Verification items for this drawing (mm, ordinates from the low corner). A direction names the side the tool comes from. Round coordinates to 2 decimals unless told otherwise and drop trailing zeros. Loops run counter-clockwise (first coordinate to the right, second up) from the corner with the lowest first, then second, coordinate; pieces in that order, holes last. Notation, with made-up numbers: (-38, -2) - (17, -2) arc R21 ccw to (17, 36) - close; hole circle Ø3 at (37, -21). An arc over 180 degrees is marked (long way). Put each result on its own line as item: value.
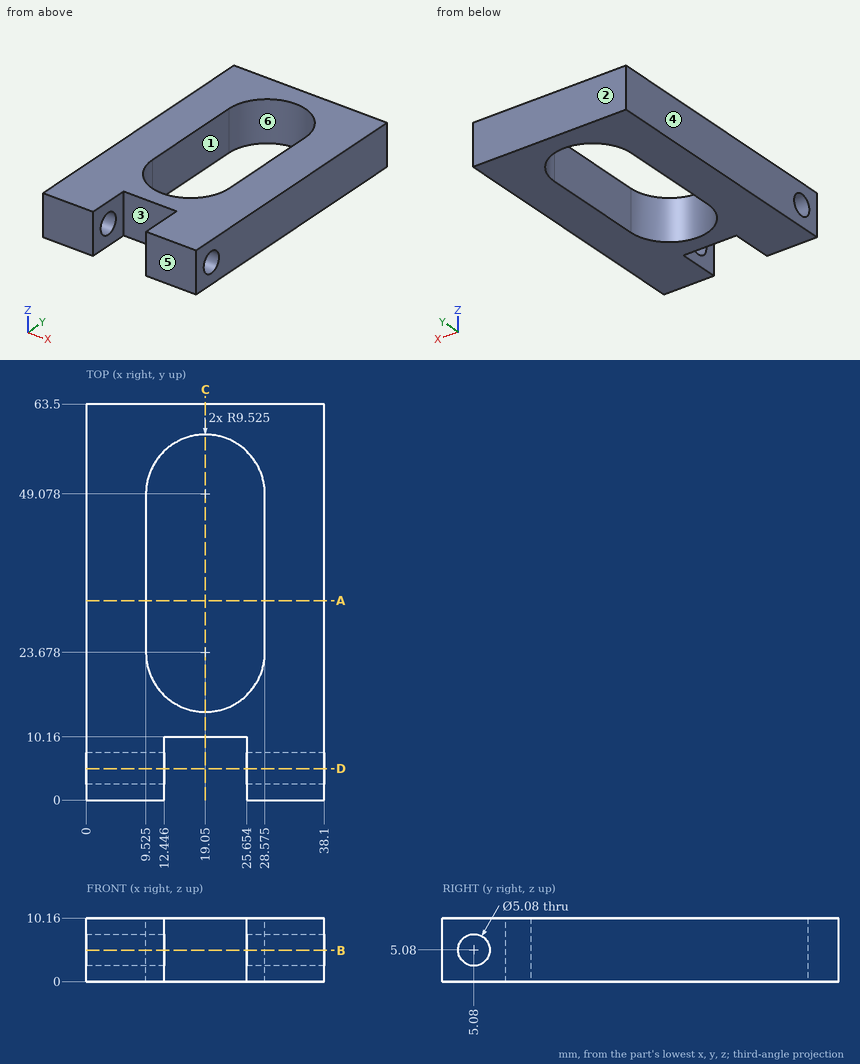
Item 1: Thickness scan on line 1 (X direction, y = 44.5, z = 4) (1 decimal); line 2 (Y direction, x = 27.5, z = 6.75) (1 decimal); line 3 (Y direction, x = 2.5, z = 5.25) (1 decimal). Record the ranges inside material, lowest first. Write a range as from..to.
Filled sheet:
line 1: 0..9.5, 28.6..38.1
line 2: 0..3.2, 7..19.3, 53.5..63.5
line 3: 0..2.5, 7.6..63.5
Item 2: Section check D-D on y = 5.08. Enter the section's corners in (x, z).
Filled sheet:
outline: (0, 0) - (12.45, 0) - (12.45, 2.54) - (0, 2.54) - close; (0, 7.62) - (12.45, 7.62) - (12.45, 10.16) - (0, 10.16) - close; (25.65, 0) - (38.1, 0) - (38.1, 2.54) - (25.65, 2.54) - close; (25.65, 7.62) - (38.1, 7.62) - (38.1, 10.16) - (25.65, 10.16) - close
Item 3: Section check A-A on y = 32. Enter the section's corners in (x, z) (1 decimal).
Filled sheet:
outline: (0, 0) - (9.5, 0) - (9.5, 10.2) - (0, 10.2) - close; (28.6, 0) - (38.1, 0) - (38.1, 10.2) - (28.6, 10.2) - close
Item 4: Tool access check on the marked faces 1, 2 and 3. Record the directions out of +Z, -Z, +X, -X, +Y, -Y that give a thin tool (end or side, any length) a straight path to the whole face; none if there is none.
Filled sheet:
face 1: +Z, -Z
face 2: +Z, -Z, +X, -X, +Y
face 3: +Z, -Z, -Y
Item 5: Go/stop test with a flat-tipped pin: pin 1 (1 mm diameter, centred on x = 13, z = 8.5, fed in from -Y). Record where the tip stops, or that it passes through.
Filled sheet:
pin 1: y = 10.16
Item 6: Release check for a two-part mould opening along Y. For the marked faces 4, 5 and 6 record: +Y half, -Y half, draft (parallel to the pull), parting line (faces both ways), or undercut.
Filled sheet:
face 4: draft
face 5: -Y half
face 6: undercut
Item 7: Section check B-B on z = 5. Count the separate pieces of the cut face and the enclosed holes in it, then the cut area to 3 significant figures.
Filled sheet:
separate pieces: 3
enclosed holes: 1
area: 1,390 mm²
Item 8: Section check C-C on x = 19.05. Enter the section's corners in (y, z).
Filled sheet:
outline: (10.16, 0) - (14.15, 0) - (14.15, 10.16) - (10.16, 10.16) - close; (58.6, 0) - (63.5, 0) - (63.5, 10.16) - (58.6, 10.16) - close
